Verification items for the finished model (mm, model axes). Face numbers are marked on the shaded views. A direction names the side the tool comes from. Give positions to 0.01 mm unless a question says otherwise; leave off trailing zeros. Write each loop counter-clockwise with the first axis right and the second up, starting at its lowest first coordinate (ties: lowest second). Pieces come first, ordered by that corner, then holes. Notation, with made-up numbers: M 83,5.25 L 111,5.25 A12 cw 111,11.25 Z; hole C -23.5,39.25 d1. An arc over 180 degrees is marked long. Answer as a JSON object with one key per item and string values.
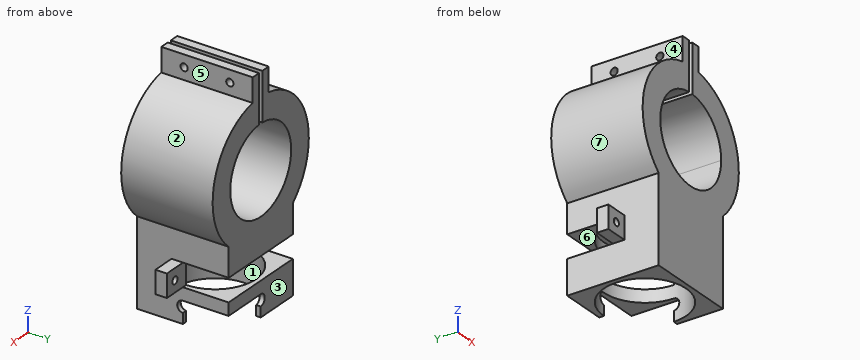
```python
from build123d import *

# Parameters (mm, degrees)
SKETCH1_R           = 19
BOSS_EXTRUDE1_DEPTH = 40
SKETCH4_W           = 40
SKETCH4_H           = 40
BOSS_EXTRUDE2_DEPTH = 30
SKETCH5_R           = 18
CUT_EXTRUDE3_DEPTH  = 30
SKETCH8_R           = 2.5
CUT_EXTRUDE5_DEPTH  = 10
SKETCH2_W           = 2
SKETCH2_H           = 21.052668078
CUT_EXTRUDE1_DEPTH  = 40
SKETCH3_R           = 1.5875
CUT_EXTRUDE2_DEPTH  = 35
SKETCH9_W           = 40
SKETCH9_H           = 10
CUT_EXTRUDE6_DEPTH  = 20
SKETCH10_W          = 10
SKETCH10_H          = 5
BOSS_EXTRUDE3_DEPTH = 10
SKETCH11_R          = 1.5875
CUT_EXTRUDE7_DEPTH  = 5
SKETCH12_W          = 20
SKETCH12_H          = 20
CUT_EXTRUDE9_DEPTH  = 2.5
CUT_EXTRUDE10_REACH = 52
SKETCH13_R          = 2.5
SKETCH14_W          = 20
SKETCH14_H          = 20
CUT_EXTRUDE11_DEPTH = 4.5


with BuildPart() as part:
    # Sketch1 → Boss-Extrude1 (new body)
    with BuildSketch(Plane(origin=(0, 0, 0), x_dir=(1, 0, 0), z_dir=(0, 1, 0))):
        with BuildLine():
            Line((5, -40), (-5, -40))
            Line((-5, -40), (-5, -29.580398915))
            ThreePointArc((-5, -29.580398915), (-28.822194814, -8.323526063), (-20, 22.360679775))
            Line((-20, 22.360679775), (-20, 30))
            Line((-20, 30), (20, 30))
            Line((20, 30), (20, 22.360679775))
            ThreePointArc((20, 22.360679775), (28.822194814, -8.323526063), (5, -29.580398915))
            Line((5, -29.580398915), (5, -40))
        make_face()
        Circle(SKETCH1_R, mode=Mode.SUBTRACT)
    extrude(amount=BOSS_EXTRUDE1_DEPTH)

    # Sketch4 → Boss-Extrude2 (add)
    with BuildSketch(Plane(origin=(0, 0, -30), x_dir=(-1, 0, 0), z_dir=(0, 0, -1))):
        with Locations((0, 20)):
            Rectangle(SKETCH4_W, SKETCH4_H)
    extrude(amount=BOSS_EXTRUDE2_DEPTH)

    # Sketch5 → Cut-Extrude3 (cut)
    with BuildSketch(Plane(origin=(0, 0, -60), x_dir=(-1, 0, 0), z_dir=(0, 0, -1))):
        with Locations((0, 20)):
            Circle(SKETCH5_R)
    extrude(amount=-CUT_EXTRUDE3_DEPTH, mode=Mode.SUBTRACT)

    # Sketch8 → Cut-Extrude5 (cut)
    with BuildSketch(Plane(origin=(0, 40, 0), x_dir=(1, 0, 0), z_dir=(0, 1, 0))):
        with Locations((0, 53)):
            Circle(SKETCH8_R)
    extrude(amount=-CUT_EXTRUDE5_DEPTH, mode=Mode.SUBTRACT)

    # Sketch2 → Cut-Extrude1 (cut)
    with BuildSketch(Plane(origin=(0, 40, 0), x_dir=(1, 0, 0), z_dir=(0, 1, 0))):
        with Locations((0, -29.5)):
            Rectangle(SKETCH2_W, SKETCH2_H)
    extrude(amount=-CUT_EXTRUDE1_DEPTH, mode=Mode.SUBTRACT)

    # Sketch3 → Cut-Extrude2 (cut)
    with BuildSketch(Plane(origin=(5, 0, 0), x_dir=(0, 0, -1), z_dir=(1, 0, 0))):
        with Locations((-34.790199458, 30)):
            Circle(SKETCH3_R)
        with Locations((-34.790199458, 10)):
            Circle(SKETCH3_R)
    extrude(amount=-CUT_EXTRUDE2_DEPTH, mode=Mode.SUBTRACT)

    # Sketch9 → Cut-Extrude6 (cut)
    with BuildSketch(Plane(origin=(0, 40, 0), x_dir=(1, 0, 0), z_dir=(0, 1, 0))):
        with Locations((0, 40)):
            Rectangle(SKETCH9_W, SKETCH9_H)
    extrude(amount=-CUT_EXTRUDE6_DEPTH, mode=Mode.SUBTRACT)

    # Sketch10 → Boss-Extrude3 (add)
    with BuildSketch(Plane.ZY.offset(20)):
        with Locations((-40, 17.5)):
            Rectangle(SKETCH10_W, SKETCH10_H)
    boss_extrude3 = extrude(amount=BOSS_EXTRUDE3_DEPTH)

    # Sketch11 → Cut-Extrude7 (cut)
    with BuildSketch(Plane(origin=(0, 20, 0), x_dir=(1, 0, 0), z_dir=(0, 1, 0))):
        with Locations((-25, 40)):
            Circle(SKETCH11_R)
    cut_extrude7 = extrude(amount=-CUT_EXTRUDE7_DEPTH, mode=Mode.SUBTRACT)

    # Mirror1: Boss-Extrude3, Cut-Extrude7 across plane
    add(boss_extrude3.mirror(Plane(origin=(0, 0, 0), x_dir=(0, 0, 1), z_dir=(1, 0, 0))))
    add(cut_extrude7.mirror(Plane(origin=(0, 0, 0), x_dir=(0, 0, 1), z_dir=(1, 0, 0))), mode=Mode.SUBTRACT)

    # Sketch12 → Cut-Extrude9 (cut, symmetric)
    with BuildSketch(Plane(origin=(0, 0, -53), x_dir=(-1, 0, 0), z_dir=(0, 0, -1))):
        with Locations((-10, 30)):
            Rectangle(SKETCH12_W, SKETCH12_H)
    extrude(amount=CUT_EXTRUDE9_DEPTH, both=True, mode=Mode.SUBTRACT)

    # Sketch13 → Cut-Extrude10 (cut, up to next)
    with BuildSketch(Plane(origin=(20, 0, 0), x_dir=(0, 0, -1), z_dir=(1, 0, 0)), mode=Mode.PRIVATE) as cut_extrude10_sk1:
        with Locations((53, 20)):
            Circle(SKETCH13_R)
    cut_extrude10_tool1 = extrude(cut_extrude10_sk1.sketch, amount=-CUT_EXTRUDE10_REACH, mode=Mode.PRIVATE) & part.part
    add(cut_extrude10_tool1.solids().sort_by_distance((20, 20, -53))[0], mode=Mode.SUBTRACT)

    # Sketch14 → Cut-Extrude11 (cut)
    with BuildSketch(Plane.XY.offset(-55.5)):
        with Locations((10, 30)):
            Rectangle(SKETCH14_W, SKETCH14_H)
    extrude(amount=-CUT_EXTRUDE11_DEPTH, mode=Mode.SUBTRACT)


solid = part.part
```
1) Section check A-A on z = -40. Record the boundary of the cut face in (x, y), and give its area (3 significant figures).
Completed:
{"outline": "M -30,15 L -26.59,15 L -26.59,20 L -30,20 Z; M -23.41,15 L -20,15 L -20,0 L 20,0 L 20,15 L 23.41,15 L 23.41,20 L 18,20 A18 cw -18,20 L -23.41,20 Z; M 26.59,15 L 30,15 L 30,20 L 26.59,20 Z", "area": "359 mm2"}
2) Go/stop test with flat-tipped pins: pin 1 (10 mm diameter, centred on x = 17.5, z = -23.5, fed in from -Y); pin 2 (17 mm diameter, centred on y = 25.5, z = 24, fed in from +X); pin 3 (2 mm diameter, centred on y = 39, z = -57, fed in from +X); pin 4 (3.5 mm diameter, centred on y = 30, z = 34.79, fed in from -X). Record where each tip stops, or that it passes through.
Completed:
{"pin 1": "stops at y = 0", "pin 2": "stops at x = 25.69", "pin 3": "stops at x = 0", "pin 4": "stops at x = -5"}
3) Thickness scan on L1, parallel to X at y = 19.5, z = -45.5; L2, parallel to X at y = 13.5, z = 0; L3, parallel to Z at x = -13.5, y = 35.5. Record the ranges inside material, lowest first.
Completed:
{"L1": "x = -20 to -17.99, 17.99 to 20", "L2": "x = -30 to -19, 19 to 30", "L3": "z = -60 to -45, -35 to -13.37, 13.37 to 26.79"}
4) Section check B-B on y = 30. Count the separate pieces of the cut face and the enclosed holes in it, and give its area (3 significant figures).
Completed:
{"separate pieces": "5", "enclosed holes": "0", "area": "1,980 mm2"}
5) Access from +Z, -Z, +X, -X, +Y, -Y to the whole of each face (thin tool, end or side, straight path). Record for the marked faces 4, 5, 6 and 7.
Completed:
{"face 4": "+Z, -X, +Y, -Y", "face 5": "+Z, +X, +Y, -Y", "face 6": "+X, -X, +Y", "face 7": "-X, +Y, -Y"}
6) Release check for a two-part mould opening along Y. For the marked faces 1, 2 and 3 record: pulls with the +Y half, pulls with the -Y half, needs draft (parallel to the pull), parting line crosses it, or undercut.
Completed:
{"face 1": "undercut", "face 2": "needs draft", "face 3": "pulls with the +Y half"}
7) Section check D-D on z = -53. Record the boundary of the cut face in (x, y).
Completed:
{"outline": "M -20,0 L 20,0 L 20,17.5 L 17.83,17.5 A18 cw long -2.5,37.83 L -2.5,40 L -20,40 Z"}
8) Section check C-C on x = 14. Record the boundary of the cut face in (y, z).
Completed:
{"outline": "M 0,-60 L 8.69,-60 L 8.69,-30 L 31.31,-30 L 31.31,-35 L 40,-35 L 40,-12.85 L 0,-12.85 Z; M 0,12.85 L 40,12.85 L 40,26.53 L 0,26.53 Z; M 31.31,-50.5 L 40,-50.5 L 40,-45 L 31.31,-45 Z"}
